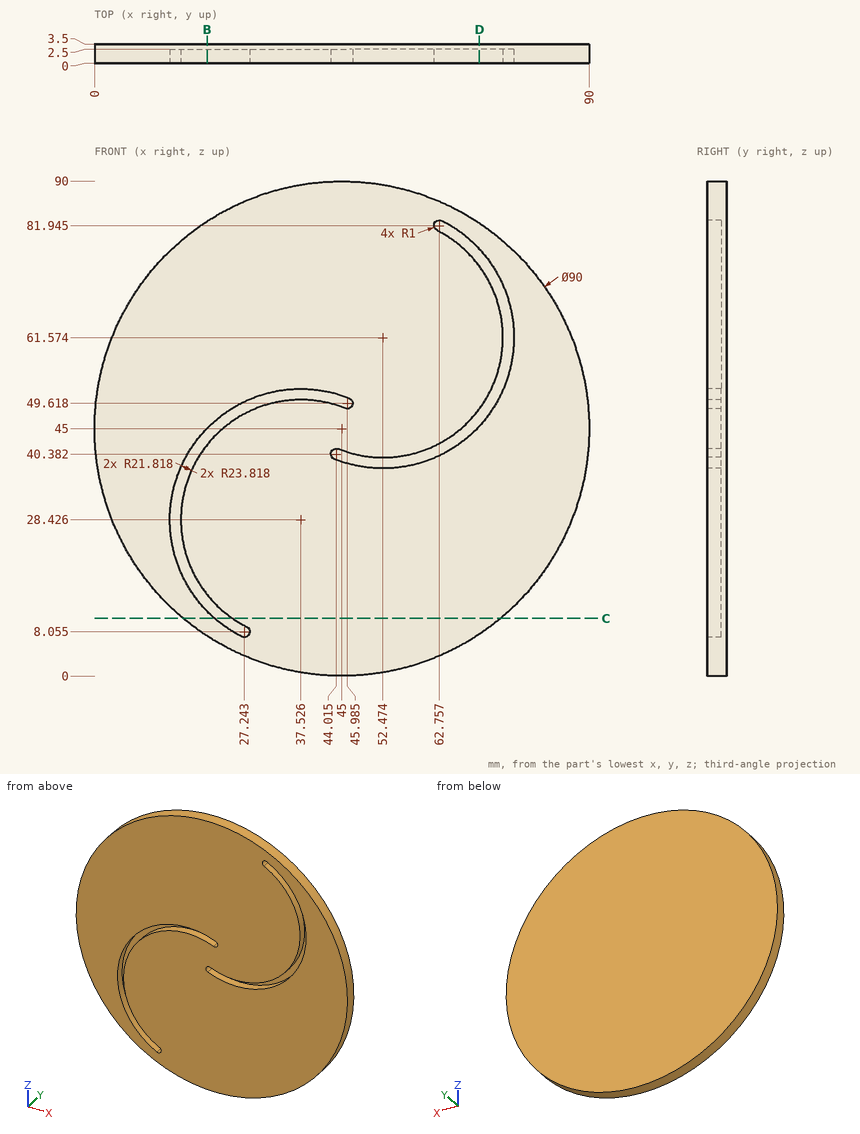
Input: dimensioned drawing with shaded views. Units: mm. Origin: part minimum x, y, z. Coordinates: 2 decimals unless noted, no trailing zeros. Order: outer loops, then holes, each group sorted by start corner. A loop starts at its lowest first (then second) coordinate and runs counter-clockwise, first axis right, second up. Notation, with made-up numbers: (77, 47.5) - (109, 47.5) arc R18 cw to (109, 51.5) - close; hole circle Ø10 at (78, 63). An arc over 180 degrees is marked (long way). Return JSON: item names as keys, results as strings. Group by question number.
1. Cut plane B-B (x = 20.5). Output: boundary loops of the cut face in (y, z) (1 decimal), plus the area to 3 significant figures.
2. Material intervals for line 1 along Z through (x, y) = (63, 1.6) (1 decimal); line 2 along X through (y, z) = (0.7, 15.5); line 3 along X through (y, z) = (1.95, 22.5) (1 decimal), sorted ascending. Write a range as [from, to].
3. Cut plane D-D (x = 70). Output: boundary loops of the cut face in (y, z) (1 decimal).
4. Cut plane C-C (z = 10.5). Output: boundary loops of the cut face in (x, y), plus the area to 3 significant figures.
Resolved:
{
 "1": {"outline": "(0, 7.3) - (3.5, 7.3) - (3.5, 82.7) - (0, 82.7) - (0, 45.1) - (2.5, 45.1) - (2.5, 42.1) - (0, 42.1) - (0, 14.8) - (2.5, 14.8) - (2.5, 11.8) - (0, 11.8) - close", "area": "249 mm²"},
 "2": {"line 1": "z = [3.8, 40.2], [42.5, 80.7], [82.9, 86.2]", "line 2": "x = [11.02, 17.52], [19.95, 78.98]", "line 3": "x = [6, 14.5], [16.5, 84]"},
 "3": {"outline": "(0, 7.6) - (3.5, 7.6) - (3.5, 82.4) - (0, 82.4) - (0, 77.7) - (2.5, 77.7) - (2.5, 74.6) - (0, 74.6) - (0, 48.6) - (2.5, 48.6) - (2.5, 45.4) - (0, 45.4) - close"},
 "4": {"outline": "(16.11, 0) - (21.84, 0) - (21.84, 2.5) - (25.09, 2.5) - (25.09, 0) - (73.89, 0) - (73.89, 3.5) - (16.11, 3.5) - close", "area": "194 mm²"}
}
